```python
from build123d import *

# Parameters (mm, degrees)
BOSS_EXTRUDE1_DEPTH            = 53.2
SKETCH2_W                      = 50
SKETCH2_H                      = 63.5
CUT_EXTRUDE1_DEPTH             = 28
F_8_0_8_DIAMETER_HOLE1_D       = 8
F_8_0_8_DIAMETER_HOLE1_DEPTH   = 1.6
F_3_7_3_7_DIAMETER_HOLE1_D     = 3.7
F_3_7_3_7_DIAMETER_HOLE2_D     = 3.7
F_3_7_3_7_DIAMETER_HOLE2_DEPTH = 1.6
F_8_0_8_DIAMETER_HOLE2_D       = 8
F_8_0_8_DIAMETER_HOLE2_DEPTH   = 1.6
F_8_0_8_DIAMETER_HOLE3_D       = 8
F_8_0_8_DIAMETER_HOLE3_DEPTH   = 1.6
FILLET1_R                      = 0.4
FILLET2_R                      = 2


with BuildPart() as part:
    # Sketch1 → Boss-Extrude1 (new body)
    with BuildSketch(Plane(origin=(26.6, 0, 0), x_dir=(0, 0, -1), z_dir=(1, 0, 0))):
        with BuildLine():
            Line((-13.5, 45), (-13.5, -1.6))
            Line((-13.5, -1.6), (13.5, -1.6))
            Line((13.5, -1.6), (13.5, 45))
            ThreePointArc((13.5, 45), (0, 58.5), (-13.5, 45))
        make_face()
    extrude(amount=-BOSS_EXTRUDE1_DEPTH)

    # Sketch2 → Cut-Extrude1 (cut, through all)
    with BuildSketch(Plane(origin=(0, 0, -13.5), x_dir=(-1, 0, 0), z_dir=(0, 0, -1))):
        with Locations((0, 31.75)):
            Rectangle(SKETCH2_W, SKETCH2_H)
    extrude(amount=-CUT_EXTRUDE1_DEPTH, mode=Mode.SUBTRACT)

    # Ø8.0 (8) Diameter Hole1
    with Locations(Plane.ZY.offset(26.6)):
        with Locations((0, 45)):
            Hole(F_8_0_8_DIAMETER_HOLE1_D / 2, depth=F_8_0_8_DIAMETER_HOLE1_DEPTH)

    # Ø3.7 (3.7) Diameter Hole1 (through all)
    with Locations(Plane.ZY.offset(26.6)):
        with Locations((0, 53), (-8, 45), (0, 37), (8, 45)):
            Hole(F_3_7_3_7_DIAMETER_HOLE1_D / 2)

    # Ø3.7 (3.7) Diameter Hole2
    with Locations(Plane(origin=(0, 0, 0), x_dir=(1, 0, 0), z_dir=(0, 1, 0))):
        with Locations((0, 8), (8, 0), (0, -8), (-8, 0)):
            Hole(F_3_7_3_7_DIAMETER_HOLE2_D / 2, depth=F_3_7_3_7_DIAMETER_HOLE2_DEPTH)

    # Ø8.0 (8) Diameter Hole2
    with Locations(Plane(origin=(0, 0, 0), x_dir=(1, 0, 0), z_dir=(0, 1, 0))):
        with Locations((0, 0)):
            Hole(F_8_0_8_DIAMETER_HOLE2_D / 2, depth=F_8_0_8_DIAMETER_HOLE2_DEPTH)

    # Ø8.0 (8) Diameter Hole3
    with Locations(Plane(origin=(26.6, 0, 0), x_dir=(0, 0, -1), z_dir=(1, 0, 0))):
        with Locations((0, 45)):
            Hole(F_8_0_8_DIAMETER_HOLE3_D / 2, depth=F_8_0_8_DIAMETER_HOLE3_DEPTH)

    # Fillet1
    fillet1_edges = [part.edges().sort_by_distance(p)[0] for p in [
        (-25, 0, 0),
        (25, 0, 0),
    ]]
    fillet(fillet1_edges, radius=FILLET1_R)

    # Fillet2
    fillet2_edges = [part.edges().sort_by_distance(p)[0] for p in [
        (-26.6, -1.6, 0),
        (26.6, -1.6, 0),
    ]]
    fillet(fillet2_edges, radius=FILLET2_R)


solid = part.part
```
Here's how the part is built. I have some questions about the finished solid (model axes, mm). A direction names the side the tool comes from. Give positions to 0.01 mm unless a question says otherwise; leave off trailing zeros. Write each loop counter-clockwise with the first axis right and the second up, starting at its lowest first coordinate (ties: lowest second). Pieces come first, ordered by that corner, then holes. Notation, with made-up numbers: M 44,-6.75 L 63,-6.75 A19 ccw 63,2.25 Z; hole C -5.5,77 d6. An arc over 180 degrees is marked long. Put each result on its own line as item: value. Start each with the question number.
Item 1: On a 3-axis mill with a long thin cutter (end or side, diameter ignored), from which of +Z, -Z, +X, -X, +Y, -Y can I reach the whole of each face in a straight line? I mean faces 1 (the cylindrical face through (25.789, 41.451, 1.846)), 2 (the flat face through (-5, 0, 0)). Say none if no direction works.
Item 2: If we section it at D-D, the plane z = 7: Write out the boundary of the cut face in (x, y).
Item 3: If we section it at B-B, the plane x = -8: Write out the boundary of the cut face in (y, z).
Item 4: I need wall thicknesses on L1, parallel to X at y = 48, z = -8; L2, parallel to Y at x = 25.9, z = 0; L3, parallel to Y at x = -9.5, z = 4.5. Which ranges of each line are inside material? Lowest first, please. Write a range as from..to.
Item 5: Thinking about a two-plate mould opening in X: for faces 3 (the cylindrical face through (26, -1.03, -0.19)), 4 (the cylindrical face through (0.867, -0.811, 3.905)), 5 (the cylindrical face through (-0.854, -0.811, 9.641)), 6 (the cylindrical face through (25.811, 43.194, 8.401)), which applies, +X half, -X half, draft (parallel to the pull), parting line (faces both ways), or undercut?
Item 6: If we section it at A-A, the plane x = 0: Write out the boundary of the cut face in (y, z), then the cut area to 3 significant figures.
Item 7: Will this pin go through, and if not, where does the flat tip stop? pin 1 (10.5 mm diameter, centred on x = 0, z = 0, fed in from +Y).
Item 8: If we section it at C-C, the plane y = 37: Write out the boundary of the cut face in (x, z).
Values:
1. face 1: +X, -X
1. face 2: +Z, -Z, +Y
2. outline: M -26.6,0.4 A2 ccw -24.6,-1.6 L -1.56,-1.6 L -1.56,0 L -24.6,0 A0.4 cw -25,0.4 L -25,43.44 L -26.6,43.44 Z; M -26.6,46.56 L -25,46.56 L -25,56.54 L -26.6,56.54 Z; M 1.56,-1.6 L 24.6,-1.6 A2 ccw 26.6,0.4 L 26.6,43.44 L 25,43.44 L 25,0.4 A0.4 cw 24.6,0 L 1.56,0 Z; M 25,46.56 L 26.6,46.56 L 26.6,56.54 L 25,56.54 Z
3. outline: M -1.6,-13.5 L 0,-13.5 L 0,-1.85 L -1.6,-1.85 Z; M -1.6,1.85 L 0,1.85 L 0,13.5 L -1.6,13.5 Z
4. L1: -26.6..-25, 25..26.6
4. L2: -1.12..35.15, 38.85..41, 49..51.15, 54.85..58.5
4. L3: -1.6..0
5. face 3: +X half
5. face 4: undercut
5. face 5: undercut
5. face 6: draft
6. outline: M -1.6,-13.5 L 0,-13.5 L 0,-9.85 L -1.6,-9.85 Z; M -1.6,-6.15 L 0,-6.15 L 0,-4 L -1.6,-4 Z; M -1.6,4 L 0,4 L 0,6.15 L -1.6,6.15 Z; M -1.6,9.85 L 0,9.85 L 0,13.5 L -1.6,13.5 Z
6. area: 18.6 mm²
7. pin 1: y = 0
8. outline: M -26.6,-13.5 L -25,-13.5 L -25,-1.85 L -26.6,-1.85 Z; M -26.6,1.85 L -25,1.85 L -25,13.5 L -26.6,13.5 Z; M 25,-13.5 L 26.6,-13.5 L 26.6,-1.85 L 25,-1.85 Z; M 25,1.85 L 26.6,1.85 L 26.6,13.5 L 25,13.5 Z
